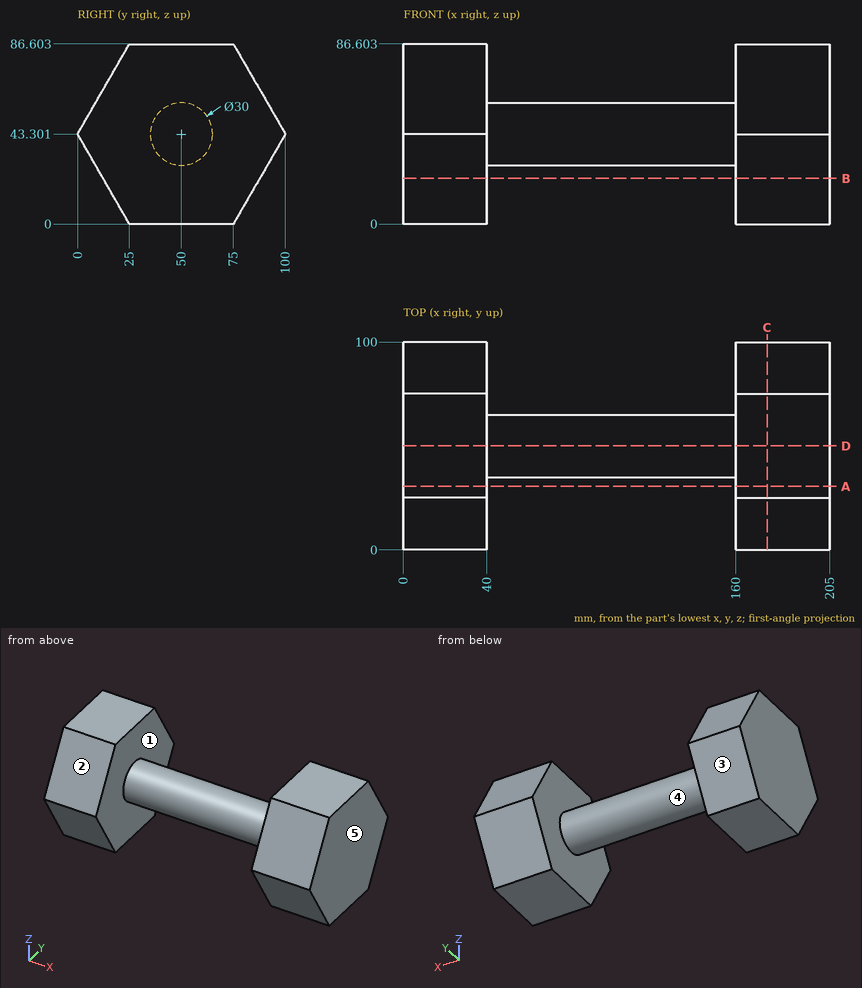
The figure shows three views and two pictorial views of one solid part (mm, origin at its lowest corner). Answer the questions. A direction names the side the tool comes from. Coordinates: 2 decimals unless noted, no trailing zeros. Write each loop counter-clockwise with the first axis right and the second up, starting at its lowest first coordinate (ties: lowest second). Pieces come first, ordered by that corner, then holes. Notation, with made-up numbers: (56, 32) -> (102, 32) arc R21 cw to (102, 46) -> close; hole circle Ø11 at (-2.75, -24.5). An arc over 180 degrees is marked (long way). Answer as a JSON object with one key per item and string values.
Q1. The part is cut by section A-A on y = 30.5. Give the vertices of the cut face in (x, z), then the cut area to 3 significant figures.
The answers:
{"outline": "(0, 0) -> (40, 0) -> (40, 86.6) -> (0, 86.6) -> close; (160, 0) -> (205, 0) -> (205, 86.6) -> (160, 86.6) -> close", "area": "7,360 mm2"}
Q2. A tool of negligible diameter and unlimited length cuts with its end or side. For the marked faces 1 and 2, from which of +Z, -Z, +X, -X, +Y, -Y can it reach the whole face along a straight path? Write none if from no direction.
The answers:
{"face 1": "none", "face 2": "+Z, +X, -X, -Y"}
Q3. A flat-ended cylindrical pin translates along its axis: pin 1 Ø4 at (x, z) = (141, 61.5) entering from -Y (1 decimal). Find the tip coordinate at first contact, or state that the pin passes through.
The answers:
{"pin 1": "passes through"}
Q4. The part is cut by section C-C on x = 175. Give the vertices of the cut face in (y, z).
The answers:
{"outline": "(0, 43.3) -> (25, 0) -> (75, 0) -> (100, 43.3) -> (75, 86.6) -> (25, 86.6) -> close"}
Q5. Consider line 1 (X direction, y = 79.5, z = 43); line 2 (Y direction, x = 197, z = 68); line 3 (Y direction, x = 52, z = 43). Determine where each line is inside the solid, lowest interval first. Write a range as [from, to].
The answers:
{"line 1": "x = [0, 40], [160, 205]", "line 2": "y = [14.26, 85.74]", "line 3": "y = [35, 65]"}
Q6. The part is cut by section D-D on y = 50. Give the vertices of the cut face in (x, z).
The answers:
{"outline": "(0, 0) -> (40, 0) -> (40, 28.3) -> (160, 28.3) -> (160, 0) -> (205, 0) -> (205, 86.6) -> (160, 86.6) -> (160, 58.3) -> (40, 58.3) -> (40, 86.6) -> (0, 86.6) -> close"}
Q7. The part is cut by section B-B on z = 22. Give the vertices of the cut face in (x, y), then the cut area to 3 significant figures.
The answers:
{"outline": "(0, 12.3) -> (40, 12.3) -> (40, 87.7) -> (0, 87.7) -> close; (160, 12.3) -> (205, 12.3) -> (205, 87.7) -> (160, 87.7) -> close", "area": "6,410 mm2"}
Q8. Determine the mould class of the marked faces 3, 4 and 5 for opening direction X: pulls with the +X half, pulls with the -X half, needs draft (parallel to the pull), parting line crosses it, or undercut.
The answers:
{"face 3": "needs draft", "face 4": "undercut", "face 5": "pulls with the +X half"}
